```python
from build123d import *

# Parameters (mm, degrees)
F1_DEPTH = 5
F3_DEPTH = 25
F5_W     = 13.2
F5_H     = 14.5
F6_DEPTH = 25


with BuildPart() as f1:
    # F0 (on Top) → F1 (new body)
    with BuildSketch(Plane.XY):
        Polygon((61.500478, 54.866199), (-52.999522, 54.866199), (-52.999522, -58.133801), (-26.674904, -80.633801), (37.000478, -80.633801), (61.500478, -54.867481), align=None)
    extrude(amount=F1_DEPTH)

    # F2 (on face) → F3 (join)
    with BuildSketch(Plane.XY.offset(5)):
        Polygon((37.000478, -80.633801), (61.500478, -54.867481), (61.500478, 54.866199), (-52.999522, 54.866199), (-52.999522, -58.133801), (-26.674904, -80.633801), align=None)
        Polygon((-47.999522, -55.829878), (-47.999522, 49.866199), (56.500478, 49.866199), (56.500478, -52.869805), (34.855248, -75.633801), (-24.829268, -75.633801), align=None, mode=Mode.SUBTRACT)
    extrude(amount=F3_DEPTH)

    # F5 (on face) → F6 (cut)
    with BuildSketch(Plane.YZ.offset(61.500478)):
        with Locations((-6.826305, 17.346862)):
            Rectangle(F5_W, F5_H)
    extrude(amount=-F6_DEPTH, mode=Mode.SUBTRACT)


solid = f1.part
```
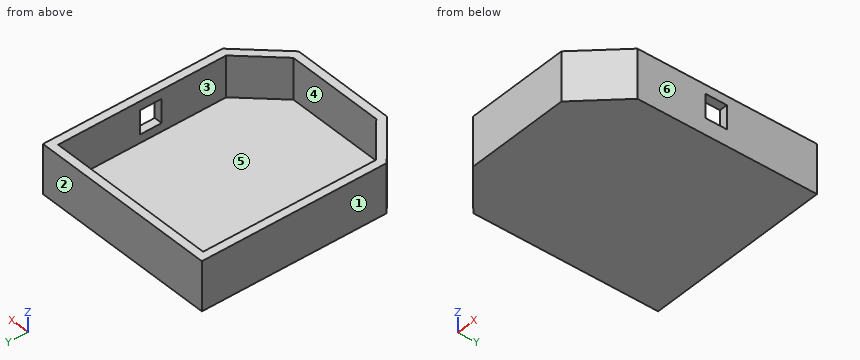
The listing builds one solid part. Answer for the finished solid, in the listing's coordinates (mm). Face numbers are marked on the shaded views. A direction names the side the tool comes from. Give positions to 0.01 mm unless a question says otherwise; leave off trailing zeros. Order: outer loops, then holes, each group sorted by start corner. A loop starts at its lowest first (then second) coordinate and runs counter-clockwise, first axis right, second up. Notation, with made-up numbers: (67.5, 83.5) -> (75.5, 83.5) arc R23 cw to (75.5, 109.5) -> close; hole circle Ø6 at (62.5, 80). An arc over 180 degrees is marked (long way). Answer as CSV lines item,"result". Start each with the question number.
Q1. A cutting plane is placed at D-D (y = 24). Determine the outline of the cut face in (x, z), then the cut area to 4 significant figures.
Q2. Which of the six approach directions +Z, -Z, +X, -X, +Y, -Y give full straight-line access (tool end or side, diameter ignored) to the marked faces 5 and 6?
Q3. Find the intervals of material crossed by L1, parallel to X at y = -42.5, z = 19.5; L2, parallel to Y at x = 33, z = 16.75; L3, parallel to X at y = -10.5, z = 21, in increasing order.
Q4. Determine the mould class of the marked faces 1, 2, 3 and 4 for opening direction Y: pulls with the +Y half, pulls with the -Y half, needs draft (parallel to the pull), parting line crosses it, or undercut.
Q5. Given pin 1 (4 mm diameter, centred on x = 60, z = 14, fed in from -Y); pin 2 (12 mm diameter, centred on x = 30, y = -49, fed in from +Z); pin 3 (8 mm diameter, centred on x = -37, z = 9, fed in from -Y), each flat-ended and moving along its own axis, determine where each tip first touches the part or whether it passes through.
Q6. A cutting plane is placed at C-C (z = 11.75). Determine the outline of the cut face in (x, y), then the cut area to 3 significant figures.
Q7. A cutting plane is placed at B-B (x = 27). Determine the outline of the cut face in (y, z), then the cut area to 4 significant figures.
Q8. A cutting plane is placed at A-A (z = 26.75). Determine the outline of the cut face in (x, y), then the cut area to 3 significant figures.
Results found:
1,outline,"(-53, 0) -> (61.5, 0) -> (61.5, 30) -> (56.5, 30) -> (56.5, 5) -> (-48, 5) -> (-48, 30) -> (-53, 30) -> close"
1,area,"822.5 mm2"
2,face 5,"+Z"
2,face 6,"+Z, -Z, +X, +Y, -Y"
3,L1,"-53 to -48, 56.5 to 61.5"
3,L2,"-80.63 to -75.63, 49.87 to 54.87"
3,L3,"-53 to -48"
4,face 1,"needs draft"
4,face 2,"pulls with the +Y half"
4,face 3,"undercut"
4,face 4,"undercut"
5,pin 1,"y = -58.55"
5,pin 2,"z = 5"
5,pin 3,"y = -75.23"
6,outline,"(-53, -58.13) -> (-26.67, -80.63) -> (37, -80.63) -> (61.5, -54.87) -> (61.5, -13.43) -> (56.5, -13.43) -> (56.5, -52.87) -> (34.86, -75.63) -> (-24.83, -75.63) -> (-48, -55.83) -> (-48, 49.87) -> (56.5, 49.87) -> (56.5, -0.23) -> (61.5, -0.23) -> (61.5, 54.87) -> (-53, 54.87) -> close"
6,area,"2,200 mm2"
7,outline,"(-80.63, 0) -> (54.87, 0) -> (54.87, 30) -> (49.87, 30) -> (49.87, 5) -> (-75.63, 5) -> (-75.63, 30) -> (-80.63, 30) -> close"
7,area,"927.5 mm2"
8,outline,"(-53, -58.13) -> (-26.67, -80.63) -> (37, -80.63) -> (61.5, -54.87) -> (61.5, 54.87) -> (-53, 54.87) -> close; hole (-48, -55.83) -> (-24.83, -75.63) -> (34.86, -75.63) -> (56.5, -52.87) -> (56.5, 49.87) -> (-48, 49.87) -> close"
8,area,"2,260 mm2"
